Can you work these out from the model? Positions are in its coordinate system, mm. A direction names the side the tool comes from. Give positions to 0.01 mm unless a question says otherwise; leave off trailing zeros. Write each loop counter-clockwise with the first axis right and the second up, starting at its lowest first coordinate (ties: lowest second). Pieces come first, ordered by that corner, then holes. Notation, with made-up numbers: (-33, -30.5) -> (10, -30.5) arc R16 ccw to (10, -8.5) -> close; hole circle Ø3 at (-18, -21.75). An arc over 180 degrees is marked (long way). Answer as CSV lines item,"result". Start each with the question number.
1. I'm going to push flat-ended pins straight in: P1, Ø2.5, axis at x = 48, y = -3.5, coming from the -Z side; P2, Ø1.3, axis at y = -4, z = 20.5, coming from the +X side; P3, Ø0.9, axis at y = -4, z = 44, coming from the -X side. Where does each tip first touch, or does it pass through?
2. I need wall thicknesses on line 1 (Z direction, x = -0.5, y = -3); line 2 (Z direction, x = 18.5, y = -0.8); line 3 (X direction, y = -1.3, z = 17.5). Which ranges of each line are inside material? Lowest first, please. Write a range as [from, to].
3. If we section it at B-B on x = 1: Write out the boundary of the cut face in (y, z), plus the area to 3 significant figures.
4. If we section it at C-C on z = 14.5: Write out the boundary of the cut face in (x, y), plus the area to 3 significant figures.
5. If we mould it in two halves opening along X, with no side actions, what happens to faces 5 (the face through (0, -3, 2)), 6 (the face through (-3, -3, 13)), 7 (the face through (43, -3, 20.25))? For each: pulls with the +X half, pulls with the -X half, needs draft (parallel to the pull), parting line crosses it, or undercut.
6. If we section it at A-A on x = 43: Write out the boundary of the cut face in (y, z).
7. On a 3-axis mill with a long thin cutter (end or side, diameter ignored), from which of +Z, -Z, +X, -X, +Y, -Y can I reach the whole of each face in a straight line? I mean faces 1 (the face through (45, -3, 24.6)), 2 (the face through (0, -3, 29)), 3 (the face through (51.4, -3, 8)), 4 (the face through (23, -3, 20.3)). Say none if no direction works.
```python
from build123d import *

# Parameters (mm, degrees)
F1_W     = 15
F1_H     = 5.4
F2_DEPTH = 5.4


with BuildPart() as f2:
    # F1 (on Front) → F2 (new body)
    with BuildSketch(Plane.XZ):
        Polygon((0, 3), (0, 0), (46, 0), (46, 3), (51.4, 3), (51.4, 13), (46, 13), (46, 21.4), (44, 21.4), (44, 20.25), (41, 20.25), (41, 21.4), (40, 21.4), (40, 23), (40, 24.6), (41, 24.6), (41, 25.75), (44, 25.75), (44, 24.6), (46, 24.6), (46, 33), (51.4, 33), (51.4, 43), (46, 43), (46, 46), (0, 46), (0, 43), (-5.4, 43), (-5.4, 33), (0, 33), (0, 24.6), (2, 24.6), (2, 25.75), (5, 25.75), (5, 24.6), (6, 24.6), (6, 23), (6, 21.4), (5, 21.4), (5, 20.25), (2, 20.25), (2, 21.4), (0, 21.4), (0, 13), (-5.4, 13), (-5.4, 3), align=None)
        with Locations((23, 23)):
            Rectangle(F1_W, F1_H, mode=Mode.SUBTRACT)
    extrude(amount=F2_DEPTH)


solid = f2.part
```
Computed values:
1,P1,"stops at z = 3"
1,P2,"stops at x = 46"
1,P3,"stops at x = 0"
2,line 1,"z = [3, 13], [33, 43]"
2,line 2,"z = [0, 20.3], [25.7, 46]"
2,line 3,"x = [0, 46]"
3,outline,"(-5.4, 0) -> (0, 0) -> (0, 21.4) -> (-5.4, 21.4) -> close; (-5.4, 24.6) -> (0, 24.6) -> (0, 46) -> (-5.4, 46) -> close"
3,area,"231 mm2"
4,outline,"(0, -5.4) -> (46, -5.4) -> (46, 0) -> (0, 0) -> close"
4,area,"248 mm2"
5,face 5,"pulls with the -X half"
5,face 6,"needs draft"
5,face 7,"undercut"
6,outline,"(-5.4, 0) -> (0, 0) -> (0, 20.25) -> (-5.4, 20.25) -> close; (-5.4, 25.75) -> (0, 25.75) -> (0, 46) -> (-5.4, 46) -> close"
7,face 1,"+X, +Y, -Y"
7,face 2,"-X, +Y, -Y"
7,face 3,"+Z, -Z, +X, +Y, -Y"
7,face 4,"+Y, -Y"
